Work out the finished part from the listing and answer in its coordinate system (mm). A direction names the side the tool comes from. Coordinates: 2 decimals unless noted, no trailing zeros. Loops run counter-clockwise (first coordinate to the right, second up) from the corner with the lowest first, then second, coordinate; pieces in that order, holes last. Notation, with made-up numbers: (-40, 66) - (-33, 66) arc R24 cw to (-33, 80) - close; hole circle Ø2 at (7.25, 81). An arc over 180 degrees is marked (long way). Write each question's results on one line, items separated by ' | '. Start each with the question number.
1. Each of these flat-tipped pins is pushed along its axis until it touches: P1, Ø8, axis at y = -9.5, z = 6.5, coming from the -X side; P2, Ø2.5, axis at y = -2, z = 21, coming from the +X side; P3, Ø4, axis at x = -5.5, z = 20.5, coming from the -Y side. Where does it stop, or does it pass through?
2. A cutting plane is placed at A-A on z = 7.5. Determine the outline of the cut face in (x, y).
3. Determine the mould class of faces 5 (the flat face through (6.24, 10.73, 19.34)), 6 (the flat face through (-21.938, 38.328, 16.457)), 7 (the flat face through (-39, -23, 15.24)) for opening direction X: released by +X, released by -X, zero draft, split by the parting line, or undercut.
4. Find the intervals of material crossed by line 1 along Y through (x, z) = (0, 19.5) (3 decimals); line 2 along Z through (x, y) = (-20, 0); line 3 along Y through (x, z) = (-15, 18.5), in increasing order. Write a range as [from, to].
5. Which of the six approach directions +Z, -Z, +X, -X, +Y, -Y give full straight-line access (tool end or side, diameter ignored) to faces 1 (the flat face through (-10.766, -6.177, 19.338)), 2 (the flat face through (38.328, 21.938, 16.457)), 3 (the flat face through (21.938, -38.328, 16.457)), 4 (the flat face through (-38.328, -21.938, 16.457))?
6. A cutting plane is placed at B-B on y = 7. State how many separate pieces and enclosed holes the cut face has, then the cut area to 3 significant figures.
from build123d import *

# Parameters (mm, degrees)
F0_R     = 45.72
F0_W     = 56.388
F0_H     = 56.388
F1_DEPTH = 15.24
F2_W     = 56.388
F2_H     = 56.388
F3_DEPTH = 10.16
F4_W     = 56.388
F4_H     = 56.388
F4_R     = 4.445
F5_DEPTH = 10.16
F6_R     = 2.413
F7_DEPTH = 31.75
F8_COUNT = 12
F9_SIZE  = 2.54


with BuildPart() as f1:
    # F0 (on Top) → F1 (new body)
    with BuildSketch(Plane.XY):
        Circle(F0_R)
        Rectangle(F0_W, F0_H, mode=Mode.SUBTRACT)
    extrude(amount=F1_DEPTH)

    # F2 (on face) → F3 (join)
    with BuildSketch(Plane.XY.offset(15.24)):
        Polygon((11.833207, 44.162129), (-11.833207, 44.162129), (-32.328922, 32.328922), (-44.162129, 11.833207), (-44.162129, -11.833207), (-32.328922, -32.328922), (-11.833207, -44.162129), (11.833207, -44.162129), (32.328922, -32.328922), (44.162129, -11.833207), (44.162129, 11.833207), (32.328922, 32.328922), align=None)
        Rectangle(F2_W, F2_H, mode=Mode.SUBTRACT)
    extrude(amount=F3_DEPTH)

    # F4 (on face) → F5 (join)
    with BuildSketch(Plane.XY.offset(25.4)):
        Rectangle(F4_W, F4_H)
        Circle(F4_R, mode=Mode.SUBTRACT)
    extrude(amount=-F5_DEPTH)

    # F9
    f9_edges = [f1.edges().sort_by_distance(p)[0] for p in [
        (38.245525, 22.081064, 25.4),
        (22.081064, 38.245525, 25.4),
        (0, 44.162129, 25.4),
        (44.162129, 0, 25.4),
        (38.245525, -22.081064, 25.4),
        (22.081064, -38.245525, 25.4),
        (0, -44.162129, 25.4),
        (-22.081064, -38.245525, 25.4),
        (-38.245525, -22.081064, 25.4),
        (-44.162129, 0, 25.4),
        (-38.245525, 22.081064, 25.4),
        (-22.081064, 38.245525, 25.4),
    ]]
    chamfer(f9_edges, length=F9_SIZE)


with BuildPart() as f7:
    # F6 (on face) → F7 (new body, symmetric)
    with BuildSketch(Plane(origin=(-38.245525, -22.081064, 0), x_dir=(0.5, -0.866025, 0), z_dir=(-0.866025, -0.5, 0))):
        with Locations((0, 19.304)):
            Circle(F6_R)
    extrude(amount=F7_DEPTH, both=True)


with BuildPart() as f8_1:
    # F8: instance of F7
    add(f7.part.rotate(Axis((0, 0, 25.4), (0, 0, 1)), 1 * 360 / F8_COUNT))


with BuildPart() as f8_2:
    # F8: instance of F7
    add(f7.part.rotate(Axis((0, 0, 25.4), (0, 0, 1)), 2 * 360 / F8_COUNT))


with BuildPart() as f8_3:
    # F8: instance of F7
    add(f7.part.rotate(Axis((0, 0, 25.4), (0, 0, 1)), 3 * 360 / F8_COUNT))


with BuildPart() as f8_4:
    # F8: instance of F7
    add(f7.part.rotate(Axis((0, 0, 25.4), (0, 0, 1)), 4 * 360 / F8_COUNT))


with BuildPart() as f8_5:
    # F8: instance of F7
    add(f7.part.rotate(Axis((0, 0, 25.4), (0, 0, 1)), 5 * 360 / F8_COUNT))


with BuildPart() as f8_6:
    # F8: instance of F7
    add(f7.part.rotate(Axis((0, 0, 25.4), (0, 0, 1)), 6 * 360 / F8_COUNT))


with BuildPart() as f8_7:
    # F8: instance of F7
    add(f7.part.rotate(Axis((0, 0, 25.4), (0, 0, 1)), 7 * 360 / F8_COUNT))


with BuildPart() as f8_8:
    # F8: instance of F7
    add(f7.part.rotate(Axis((0, 0, 25.4), (0, 0, 1)), 8 * 360 / F8_COUNT))


with BuildPart() as f8_9:
    # F8: instance of F7
    add(f7.part.rotate(Axis((0, 0, 25.4), (0, 0, 1)), 9 * 360 / F8_COUNT))


with BuildPart() as f8_10:
    # F8: instance of F7
    add(f7.part.rotate(Axis((0, 0, 25.4), (0, 0, 1)), 10 * 360 / F8_COUNT))


with BuildPart() as f8_11:
    # F8: instance of F7
    add(f7.part.rotate(Axis((0, 0, 25.4), (0, 0, 1)), 11 * 360 / F8_COUNT))


with BuildPart() as f1_1:
    add(f1.part)

    # F10: cut F8_2, F8_1, F7, F8_11, F8_10, F8_9, F8_8, F8_7, F8_6, F8_5, F8_4, F8_3
    add(f8_2.part, mode=Mode.SUBTRACT)
    add(f8_1.part, mode=Mode.SUBTRACT)
    add(f7.part, mode=Mode.SUBTRACT)
    add(f8_11.part, mode=Mode.SUBTRACT)
    add(f8_10.part, mode=Mode.SUBTRACT)
    add(f8_9.part, mode=Mode.SUBTRACT)
    add(f8_8.part, mode=Mode.SUBTRACT)
    add(f8_7.part, mode=Mode.SUBTRACT)
    add(f8_6.part, mode=Mode.SUBTRACT)
    add(f8_5.part, mode=Mode.SUBTRACT)
    add(f8_4.part, mode=Mode.SUBTRACT)
    add(f8_3.part, mode=Mode.SUBTRACT)


solid = f1_1.part
Values:
1) P1: x = -45.39 | P2: x = 44.16 | P3: y = -44.16
2) outline: circle Ø91.44 at (0, 0); hole (-28.19, -28.19) - (28.19, -28.19) - (28.19, 28.19) - (-28.19, 28.19) - close
3) face 5: undercut | face 6: released by -X | face 7: zero draft
4) line 1: [-12.412, -4.445], [4.445, 12.412] | line 2: [15.24, 16.89], [21.72, 25.4] | line 3: [-42.33, -30.53], [-21.43, -11.29], [-6.03, -2.28], [2.28, 6.03], [11.29, 21.43], [30.53, 42.33]
5) face 1: none | face 2: +Z, +X, +Y | face 3: +Z, +X, -Y | face 4: +Z, -X, -Y
6) separate pieces: 1 | enclosed holes: 2 | area: 1,350 mm^2
